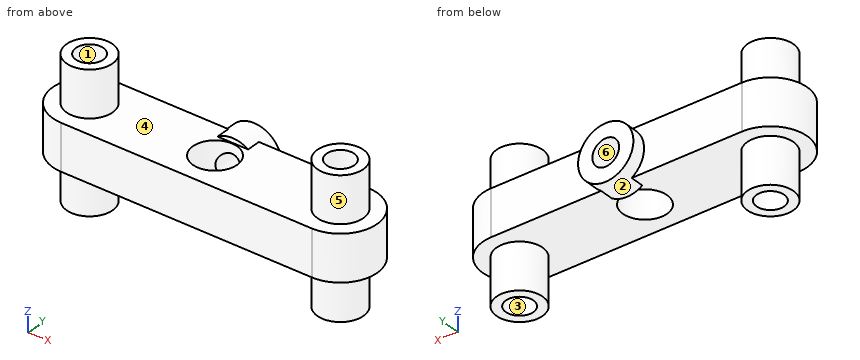
```python
from build123d import *

# Parameters (mm, degrees)
SKETCH1_R           = 2.4
BOSS_EXTRUDE1_DEPTH = 5
SKETCH5_R           = 3
BOSS_EXTRUDE3_DEPTH = 1.5
SKETCH6_R           = 1.45
CUT_EXTRUDE4_DEPTH  = 9
SKETCH2_R           = 1.45
CUT_EXTRUDE3_DEPTH  = 4
SKETCH7_R           = 2.5
SKETCH7_R_2         = 1.5
BOSS_EXTRUDE4_DEPTH = 5


with BuildPart() as part:
    # Sketch1 → Boss-Extrude1 (new body)
    with BuildSketch(Plane.XY):
        with BuildLine():
            Line((0, 4), (27.2, 4))
            ThreePointArc((27.2, 4), (31.2, 0), (27.2, -4))
            Line((27.2, -4), (0, -4))
            ThreePointArc((0, -4), (-4, 0), (0, 4))
        make_face()
        with Locations((13.6, 0)):
            Circle(SKETCH1_R, mode=Mode.SUBTRACT)
    extrude(amount=BOSS_EXTRUDE1_DEPTH)

    # Sketch5 → Boss-Extrude3 (add, symmetric)
    with BuildSketch(Plane(origin=(0, 4, 0), x_dir=(1, 0, 0), z_dir=(0, 1, 0))):
        with Locations((13.6, -2.5)):
            Circle(SKETCH5_R)
    extrude(amount=BOSS_EXTRUDE3_DEPTH, both=True)

    # Sketch6 → Cut-Extrude4 (cut)
    with BuildSketch(Plane.XY.offset(5)):
        with Locations((27.2, 0)):
            Circle(SKETCH6_R)
        Circle(SKETCH6_R)
    cut_extrude4 = extrude(amount=-CUT_EXTRUDE4_DEPTH, mode=Mode.SUBTRACT)

    # Sketch2 → Cut-Extrude3 (cut, symmetric)
    with BuildSketch(Plane(origin=(0, 4, 0), x_dir=(1, 0, 0), z_dir=(0, 1, 0))):
        with Locations((13.6, -2.5)):
            Circle(SKETCH2_R)
    extrude(amount=CUT_EXTRUDE3_DEPTH, both=True, mode=Mode.SUBTRACT)

    # Sketch7 → Boss-Extrude4 (add)
    with BuildSketch(Plane.XY.offset(5)):
        with Locations((27.2, 0)):
            Circle(SKETCH7_R)
        with Locations((27.2, 0)):
            Circle(SKETCH7_R_2, mode=Mode.SUBTRACT)
        Circle(SKETCH7_R)
        Circle(SKETCH7_R_2, mode=Mode.SUBTRACT)
    boss_extrude4 = extrude(amount=BOSS_EXTRUDE4_DEPTH)

    # Mirror1: Cut-Extrude4, Boss-Extrude4 across plane
    add(cut_extrude4.mirror(Plane(origin=(0, 0, 2.5), x_dir=(1, 0, 0), z_dir=(0, 0, -1))), mode=Mode.SUBTRACT)
    add(boss_extrude4.mirror(Plane(origin=(0, 0, 2.5), x_dir=(1, 0, 0), z_dir=(0, 0, -1))))


solid = part.part
```
Can you work these out from the model? Positions are in its coordinate system, mm. Face numbers are marked on the shaded views. A direction names the side the tool comes from. Coordinates: 2 decimals unless noted, no trailing zeros. Loops run counter-clockwise (first coordinate to the right, second up) from the corner with the lowest first, then second, coordinate; pieces in that order, holes last.
1) Imagine slicing it at A-A on x = 13.6. List the corners of the cut face in (y, z) for me, plus the area to 3 significant figures.
2) Imagine slicing it at D-D on z = -3. List the corners of the cut face in (x, y) for me, plus the area to 3 significant figures.
3) I need wall thicknesses on probe 1 along Y at (x, z) = (27.2, -3.15); probe 2 along X at (y, z) = (-0.25, 8); probe 3 along X at (y, z) = (0.5, 1.25). Which ranges of each line are inside material? Lowest first, please.
4) Thinking about a two-plate mould opening in Z: for the marked faces 4, 5 and 6, which applies, pulls with the +Z half, pulls with the -Z half, needs draft (parallel to the pull), parting line crosses it, or undercut?
5) Imagine slicing it at C-C on y = 0. State how many separate pieces and enclosed holes the cut face has, plus the area to 3 significant figures.
6) For pin 1 (3 mm diameter, centred on x = 5, z = -3, fed in from +Y); pin 2 (1.5 mm diameter, centred on x = 9, z = 1.5, fed in from +Y); pin 3 (2.5 mm diameter, centred on x = 20, y = 0, fed in from -Z); pin 4 (5 mm diameter, centred on x = 17, y = 2.5, fed in from +Z), each with a flat end and sliding along its axis, tell me the tip position at first contact or that it passes through.
7) Which directions (+Z, -Z, +X, -X, +Y, -Y) give clear straight access to the entire face, cutting with the end or side of a thin tool? Please do the marked faces 1, 2 and 3.
8) Imagine slicing it at B-B on z = 2.5. List the corners of the cut face in (x, y) for me.
Completed:
1. outline: (-4, 0) - (-2.4, 0) - (-2.4, 5) - (-4, 5) - close; (2.4, 0) - (2.5, 0) - (2.5, -0.5) - (5.5, -0.5) - (5.5, 1.05) - (2.4, 1.05) - close; (2.4, 3.95) - (5.5, 3.95) - (5.5, 5.5) - (2.5, 5.5) - (2.5, 5) - (2.4, 5) - close
1. area: 17.5 mm2
2. outline: circle Ø5 at (0, 0); circle Ø5 at (27.2, 0); hole circle Ø3 at (0, 0); hole circle Ø3 at (27.2, 0)
2. area: 25.1 mm2
3. probe 1: y = -2.5 to -1.5, 1.5 to 2.5
3. probe 2: x = -2.49 to -1.48, 1.48 to 2.49, 24.71 to 25.72, 28.68 to 29.69
3. probe 3: x = -3.97 to -1.36, 1.36 to 11.25, 15.95 to 25.84, 28.56 to 31.17
4. face 4: pulls with the +Z half
4. face 5: needs draft
4. face 6: undercut
5. separate pieces: 4
5. enclosed holes: 0
5. area: 163 mm2
6. pin 1: passes through
6. pin 2: stops at y = 4
6. pin 3: stops at z = 0
6. pin 4: stops at z = 5.36
7. face 1: +Z
7. face 2: +Y
7. face 3: -Z
8. outline: (0, -4) - (27.2, -4) arc R4 ccw to (27.2, 4) - (16.6, 4) - (16.6, 5.5) - (15.05, 5.5) - (15.05, 1.91) arc R2.4 cw (long way) to (12.15, 1.91) - (12.15, 5.5) - (10.6, 5.5) - (10.6, 4) - (0, 4) arc R4 ccw to start; hole circle Ø2.9 at (0, 0); hole circle Ø2.9 at (27.2, 0)
